Solid Edge part; units mm, degrees
sketch "Sketch1" plane through (0, 0, 0) normal (0, 0, 1) x (1, 0, 0)
  line L0 (40, -11) -> (-40, -11)
  line L1 (-40, -11) -> (-40, 11)
  line L2 (-40, 11) -> (40, 11)
  line L3 (40, 11) -> (40, -11)
  dimension "D1" = 40
  dimension "D2" = 40
extrude "Protrusion1" add sketch "Sketch1" along normal blind 5.5
hole "Hole_1" at (37, 8, 5.5) direction (0, 0, -1) diameter 2 end through all
hole "Hole1" at (37, -8, 5.5) direction (0, 0, -1) diameter 2 end through all
hole "Hole2" at (-37, 8, 5.5) direction (0, 0, -1) diameter 2 end through all
hole "Hole3" at (-37, -8, 5.5) direction (0, 0, -1) diameter 2 end through all
hole "Hole4" at (-29, 0, 5.5) direction (0, 0, -1) diameter 2 end through all
hole "Hole5" at (29, 0, 5.5) direction (0, 0, -1) diameter 2 end through all
fillet "Round_1" radius 2 3 edges at (-40, 11, 2.75) (-40, -11, 2.75) (40, -11, 2.75)
fillet "Round_2" radius 2 1 edges at (40, 11, 2.75)
properties material "木材, アッシュ"
The listing builds one solid part. Answer for the finished solid, in the listing's coordinates (mm). Round coordinates to 2 decimals unless told otherwise and drop trailing zeros. Write each loop counter-clockwise with the first axis right and the second up, starting at its lowest first coordinate (ties: lowest second). Pieces come first, ordered by that corner, then holes. Notation, with made-up numbers: (-32.5, 5.25) -> (-1.5, 5.25) arc R36 cw to (-1.5, 40.25) -> close; hole circle Ø2 at (3, 17). An arc over 180 degrees is marked (long way). Use CSV: the item, a comma, the result in double quotes. Start each with the question number.
(1) Consider L1, parallel to X at y = 8, z = 1.65; L2, parallel to Y at x = 37, z = 1.4; L3, parallel to X at y = 0, z = 4.3. Determine where each line is inside the solid, lowest interval first. Write a range as from..to.
(2) Section A-A on x = 29 is taken. Give the vertices of the cut face in (y, z), then the cut area to 3 significant figures.
(3) Each of these flat-tipped pins is pushed along its axis until it touches: pin 1 (2.5 mm diameter, centred on x = 29, y = 0, fed in from +Z); pin 2 (1.8 mm diameter, centred on x = -37, y = 8, fed in from -Z) (3 decimals). Where does it stop, or does it pass through?
(4) Section B-B on y = -8 is taken. Give the vertices of the cut face in (x, z), then the cut area to 3 significant figures.
(5) The mould has two halves that part along Y. Classify faces 1 (the face through (1, 0, 0)), 2 (the face through (39.43, 10.4, 2.79)), 3 (the face through (-28, 0, 3)), 4 (the face through (-39.43, -10.4, 2.79)): released by +Y, released by -Y, zero draft, split by the parting line, or undercut.
A:
1,L1,"x = -40..-38, -36..36, 38..40"
1,L2,"y = -11..-9, -7..7, 9..11"
1,L3,"x = -40..-30, -28..28, 30..40"
2,outline,"(-11, 0) -> (-1, 0) -> (-1, 5.5) -> (-11, 5.5) -> close; (1, 0) -> (11, 0) -> (11, 5.5) -> (1, 5.5) -> close"
2,area,"110 mm²"
3,pin 1,"stops at z = 5.5"
3,pin 2,"passes through"
4,outline,"(-40, 0) -> (-38, 0) -> (-38, 5.5) -> (-40, 5.5) -> close; (-36, 0) -> (36, 0) -> (36, 5.5) -> (-36, 5.5) -> close; (38, 0) -> (40, 0) -> (40, 5.5) -> (38, 5.5) -> close"
4,area,"418 mm²"
5,face 1,"zero draft"
5,face 2,"released by +Y"
5,face 3,"undercut"
5,face 4,"released by -Y"
